Answer from the drawing. Dimensions are ordinates in mm from the lowest x, y and z of the part. A direction names the side the tool comes from. Coordinates: 2 decimals unless noted, no trailing zeros. Write each loop counter-clockwise with the first axis right and the second up, starting at its lowest first coordinate (ties: lowest second). Pieces come first, ordered by that corner, then holes.
(1) The part is cut by section C-C, the plane x = 23.5. Determine the outline of the cut face in (y, z).
(2) Given pin 1 (2 mm diameter, centred on x = 57.5, z = 33, fed in from -Y); pin 2 (10 mm diameter, centred on x = 100.5, z = 7.5, fed in from -Y); pin 3 (4 mm diameter, centred on x = 48.5, z = 17.5, fed in from +Y), each flat-ended and moving along its own axis, determine where each tip first touches the part or whether it passes through.
(3) The part is cut by section B-B, the plane y = 31.75. Determine the outline of the cut face in (x, z), and give its area (3 significant figures).
(4) The part is cut by section A-A, the plane z = 40. State how many separate pieces and enclosed holes the cut face has, and give its area (3 significant figures).
(5) Which of the six approach directions +Z, -Z, +X, -X, +Y, -Y give full straight-line access (tool end or side, diameter ignored) to the marked faces 1, 2 and 3?
(6) Straight lines are drawn through the part: line 1 along X through (y, z) = (31, 41) (1 decimal); line 2 along X through (y, z) = (36, 31) (1 decimal); line 3 along Y through (x, z) = (44, 20.5). For each, find the intervals that lie inside material, in ascending order.
(7) Determine the mould class of the marked faces 4, 5 and 6 for opening direction X: pulls with the +X half, pulls with the -X half, needs draft (parallel to the pull), parting line crosses it, or undercut.
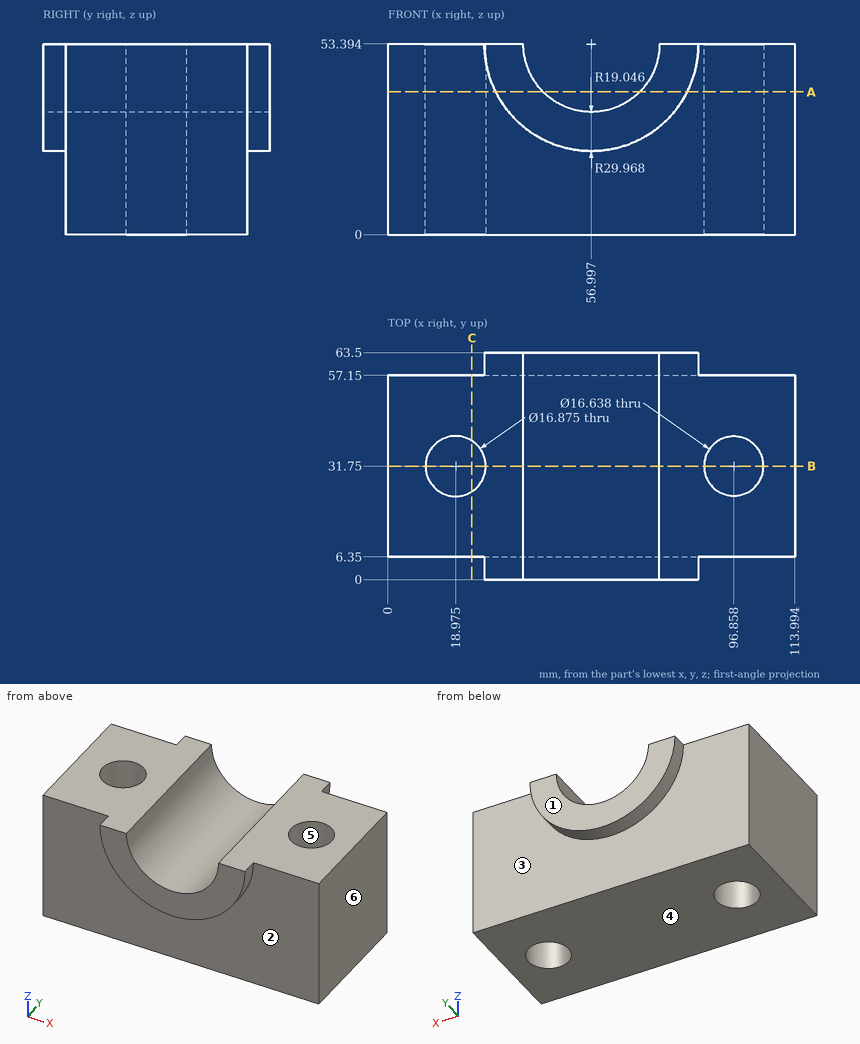
Computed:
1. outline: (6.35, 0) - (24.63, 0) - (24.63, 53.39) - (6.35, 53.39) - close; (38.87, 0) - (57.15, 0) - (57.15, 53.39) - (38.87, 53.39) - close
2. pin 1: stops at y = 0
2. pin 2: stops at y = 6.35
2. pin 3: stops at y = 57.15
3. outline: (0, 0) - (10.54, 0) - (10.54, 53.39) - (0, 53.39) - close; (27.41, 0) - (88.54, 0) - (88.54, 53.39) - (76.04, 53.39) arc R19.05 cw to (37.95, 53.39) - (27.41, 53.39) - close; (105.18, 0) - (113.99, 0) - (113.99, 53.39) - (105.18, 53.39) - close
3. area: 3,730 mm2
4. separate pieces: 2
4. enclosed holes: 2
4. area: 4,310 mm2
5. face 1: +Z, -Z, +X, -X, +Y
5. face 2: -Z, -Y
5. face 3: -Z, +Y
6. line 1: x = 0 to 10.6, 27.4 to 42.5, 71.5 to 88.6, 105.1 to 114
6. line 2: x = 0 to 11.7, 26.3 to 89.7, 104 to 114
6. line 3: y = 6.35 to 57.15
7. face 4: needs draft
7. face 5: undercut
7. face 6: pulls with the +X half
